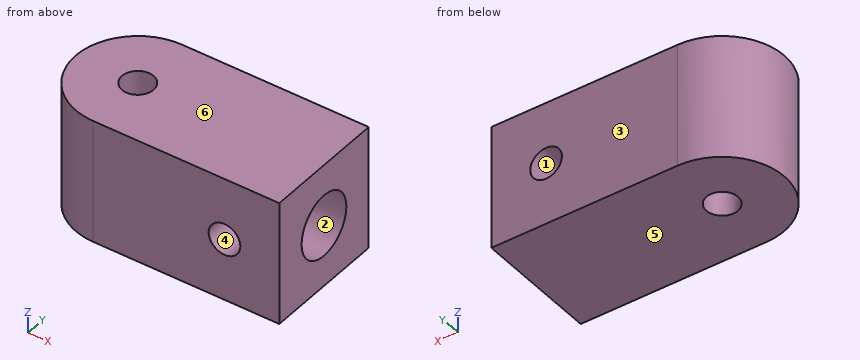
from build123d import *

# Parameters (mm, degrees)
SKETCH_R        = 2.55
PAD_DEPTH       = 20
SKETCH001_R     = 5
POCKET_DEPTH    = 15
SKETCH003_R     = 2.55
POCKET001_DEPTH = 20.001


with BuildPart() as part:
    # Sketch → Pad (new body)
    with BuildSketch(Plane.XY):
        with BuildLine():
            Line((-30, 10), (0, 10))
            Line((0, 10), (0, -10))
            Line((0, -10), (-30, -10))
            ThreePointArc((-30, 10), (-40, 0), (-30, -10))
        make_face()
        with Locations((-30, 0)):
            Circle(SKETCH_R, mode=Mode.SUBTRACT)
    extrude(amount=PAD_DEPTH)

    # Sketch001 (on Face2 of Pad) → Pocket (cut)
    with BuildSketch(Plane.YZ):
        with Locations((0, 10)):
            Circle(SKETCH001_R)
    extrude(amount=-POCKET_DEPTH, mode=Mode.SUBTRACT)

    # Sketch003 (on Face6 of Pocket) → Pocket001 (cut, through all)
    with BuildSketch(Plane.XZ.offset(10)):
        with Locations((-8.827239, 10)):
            Circle(SKETCH003_R)
    extrude(amount=-POCKET001_DEPTH, mode=Mode.SUBTRACT)


solid = part.part
Check sheet for the modelled part. Datum: model origin and axes. Units: mm. Face numbers are marked on the shaded views. A direction names the side the tool comes from. Give positions to 0.01 mm unless a question says otherwise; leave off trailing zeros. Loops run counter-clockwise (first coordinate to the right, second up) from the corner with the lowest first, then second, coordinate; pieces in that order, holes last. Notation, with made-up numbers: M -9.5,-5.75 L 1.5,-5.75 A25 ccw 1.5,9.25 Z; hole C -2.75,46.5 d4. An arc over 180 degrees is marked long. Return JSON: item names as keys, results as strings. Group by question number.
1. Cross-section at B-B on y = 0. Record the boundary of the cut face in (x, z), plus the area to 3 significant figures.
2. Cross-section at A-A on z = 10. Record the boundary of the cut face in (x, y), plus the area to 3 significant figures.
3. Cross-section at D-D on z = 6.5. Record the boundary of the cut face in (x, y), plus the area to 3 significant figures.
4. Tool access check on the marked faces 1 and 2. Record the directions out of +Z, -Z, +X, -X, +Y, -Y that give a thin tool (end or side, any length) a straight path to the whole face; none if there is none.
5. Cross-section at C-C on x = -9. Record the boundary of the cut face in (y, z).
6. Mould release check, pull along Z, two halves, no side actions. Record for the marked faces 3, 4, 5 and 6: released by +Z, released by -Z, zero draft, split by the parting line, or undercut.
7. Go/stop test with flat-tipped pins: pin 1 (4 mm diameter, centred on x = -8.83, z = 10, fed in from -Y); pin 2 (3 mm diameter, centred on y = 0.5, z = 9.5, fed in from +X). Record where each tip stops, or that it passes through.
8. Thickness scan on L1, parallel to Y at x = -30, z = 2.75; L2, parallel to Z at x = -6.25, y = 0; L3, parallel to X at y = -2, z = 12.5. Record the ranges inside material, lowest first.
Return value:
{
 "1": {"outline": "M -40,0 L -32.55,0 L -32.55,20 L -40,20 Z; M -27.45,0 L 0,0 L 0,5 L -15,5 L -15,15 L 0,15 L 0,20 L -27.45,20 Z", "area": "548 mm^2"},
 "2": {"outline": "M -30,-10 L -11.38,-10 L -11.38,-5 L -15,-5 L -15,5 L -11.38,5 L -11.38,10 L -30,10 A10 ccw Z; M -6.28,-10 L 0,-10 L 0,-5 L -6.28,-5 Z; M -6.28,5 L 0,5 L 0,10 L -6.28,10 Z; hole C -30,0 d5.1", "area": "536 mm^2"},
 "3": {"outline": "M -30,-10 L 0,-10 L 0,-3.57 L -15,-3.57 L -15,3.57 L 0,3.57 L 0,10 L -30,10 A10 ccw Z; hole C -30,0 d5.1", "area": "630 mm^2"},
 "4": {"face 1": "+Y, -Y", "face 2": "+X"},
 "5": {"outline": "M -10,0 L 10,0 L 10,7.46 L 4.3,7.46 A5 cw -4.3,7.46 L -10,7.46 Z; M -10,12.54 L -4.3,12.54 A5 cw 4.3,12.54 L 10,12.54 L 10,20 L -10,20 Z"},
 "6": {"face 3": "zero draft", "face 4": "undercut", "face 5": "released by -Z", "face 6": "released by +Z"},
 "7": {"pin 1": "through", "pin 2": "x = -15"},
 "8": {"L1": "-10 to -2.55, 2.55 to 10", "L2": "0 to 5, 15 to 20", "L3": "-39.8 to -31.58, -28.42 to -15"}
}
